```python
from build123d import *

# Parameters (mm, degrees)
SKETCH1_R           = 2.125
SKETCH1_W           = 4
SKETCH1_H           = 20
BOSS_EXTRUDE2_DEPTH = 4


with BuildPart() as part:
    # Sketch1 → Boss-Extrude2 (new body)
    with BuildSketch(Plane(origin=(0, 0, 0), x_dir=(1, 0, 0), z_dir=(0, 1, 0))):
        Polygon((64, 0), (64, -4), (84, -4), (84, 0), (144, 0), (144, -4), (164, -4), (164, 0), (184, 0), (184, -4), (204, -4), (204, 0), (228, 0), (228, 36), (0, 36), (0, 0), (24, 0), (24, -4), (44, -4), (44, 0), align=None)
        with Locations((4, 3.5)):
            Circle(SKETCH1_R, mode=Mode.SUBTRACT)
        with Locations((28.5, 3.5)):
            Circle(SKETCH1_R, mode=Mode.SUBTRACT)
        with Locations((199.5, 3.5)):
            Circle(SKETCH1_R, mode=Mode.SUBTRACT)
        with Locations((224, 3.5)):
            Circle(SKETCH1_R, mode=Mode.SUBTRACT)
        with Locations((12, 20)):
            Rectangle(SKETCH1_W, SKETCH1_H, mode=Mode.SUBTRACT)
        with Locations((4, 28)):
            Circle(SKETCH1_R, mode=Mode.SUBTRACT)
        with Locations((28.5, 28)):
            Circle(SKETCH1_R, mode=Mode.SUBTRACT)
        with Locations((216, 20)):
            Rectangle(SKETCH1_W, SKETCH1_H, mode=Mode.SUBTRACT)
        with Locations((199.5, 28)):
            Circle(SKETCH1_R, mode=Mode.SUBTRACT)
        with Locations((224, 28)):
            Circle(SKETCH1_R, mode=Mode.SUBTRACT)
    extrude(amount=BOSS_EXTRUDE2_DEPTH)


solid = part.part
```
Read the model definition and answer for the solid it produces. Units are mm, in the model's axes. A direction names the side the tool comes from. Give positions to 0.01 mm unless a question says otherwise; leave off trailing zeros. Loops run counter-clockwise (first coordinate to the right, second up) from the corner with the lowest first, then second, coordinate; pieces in that order, holes last.
Item 1: The mould has two halves that part along X. Classify faces 4 (the flat face through (112, 0, -16)), 5 (the flat face through (214, 2, -20)), 6 (the flat face through (0, 2, -18)): released by +X, released by -X, zero draft, split by the parting line, or undercut.
Item 2: The part is cut by section C-C (y = 3). Give the number of separate pieces and of enclosed holes in the cut face, and give its area (3 significant figures).
Item 3: The part is cut by section A-A (x = 4). Write down the section's boundary in (y, z) (3 decimals), and give its area (3 significant figures).
Item 4: The part is cut by section B-B (z = -23). Write down the section's boundary in (x, y), and give its area (3 significant figures).
Item 5: The part is cut by section D-D (x = 108.5). Write down the section's boundary in (y, z), and give its area (3 significant figures).
Item 6: For faces 1 (the flat face through (44, 2, 2)), 2 (the flat face through (12, 2, -30)), 3 (the flat face through (112, 4, -16)), determine the directions among +Z, -Z, +X, -X, +Y, -Y from which every point of the face is accessible in a straight line to the end or side of a thin tool.
Item 7: Each of these flat-tipped pins is pushed along its axis until it touches: pin 1 Ø1.2 at (y, z) = (2, 1.5) entering from -X; pin 2 Ø2 at (x, y) = (13, 1.5) entering from +Z. Where does it stop, or does it pass through?
Item 8: Find the intervals of material crossed by line 1 along Z through (x, y) = (28.5, 0.95) (3 decimals); line 2 along Z through (x, y) = (224, 2.8) (3 decimals); line 3 along X through (y, z) = (2.05, -3.5) (3 decimals), in increasing order.
Taken from the geometry:
1. face 4: zero draft
1. face 5: undercut
1. face 6: released by -X
2. separate pieces: 1
2. enclosed holes: 10
2. area: 8,250 mm2
3. outline: (0, -36) - (4, -36) - (4, -30.125) - (0, -30.125) - close; (0, -25.875) - (4, -25.875) - (4, -5.625) - (0, -5.625) - close; (0, -1.375) - (4, -1.375) - (4, 0) - (0, 0) - close
3. area: 110 mm2
4. outline: (0, 0) - (10, 0) - (10, 4) - (0, 4) - close; (14, 0) - (214, 0) - (214, 4) - (14, 4) - close; (218, 0) - (228, 0) - (228, 4) - (218, 4) - close
4. area: 880 mm2
5. outline: (0, -36) - (4, -36) - (4, 0) - (0, 0) - close
5. area: 144 mm2
6. face 1: +Z, +Y, -Y
6. face 2: +Y, -Y
6. face 3: +Z, -Z, +X, -X, +Y
7. pin 1: stops at x = 24
7. pin 2: stops at z = 0
8. line 1: z = -36 to -30.125, -25.875 to -5.625, -1.375 to 4
8. line 2: z = -36 to -30.125, -25.875 to -5.625, -1.375 to 0
8. line 3: x = 0 to 1.875, 6.125 to 26.375, 30.625 to 197.375, 201.625 to 221.875, 226.125 to 228
